Read the model definition and answer for the solid it produces. Units are mm, in the model's axes. Face numbers are marked on the shaded views. A direction names the side the tool comes from. Coordinates: 2 decimals unless noted, no trailing zeros. Order: outer loops, then holes, each group sorted by start corner. A loop starts at its lowest first (then second) coordinate and runs counter-clockwise, first axis right, second up. Notation, with made-up numbers: M 14,-35.5 L 73,-35.5 A10 ccw 73,-26.5 Z; hole C -31,37.25 d4. An arc over 180 degrees is marked long. Write each question's results on one line, items separated by ' | '.
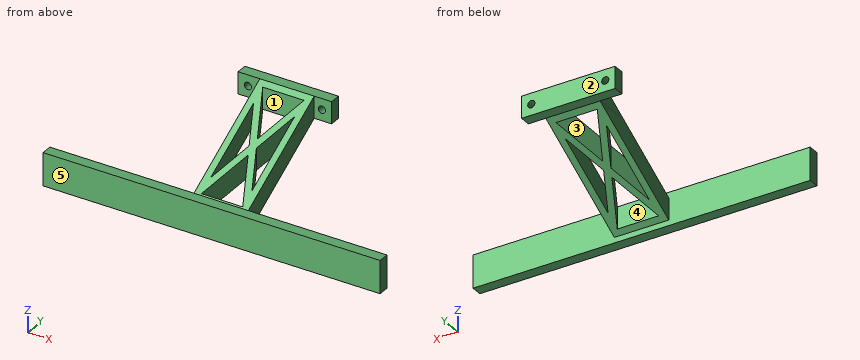
Autodesk Inventor part; units mm, degrees
ref_plane "YZ Plane" through (0, 0, 0) normal (1, 0, 0) x (0, 1, 0)
ref_plane "XZ Plane" through (0, 0, 0) normal (0, 1, 0) x (-1, 0, 0)
ref_plane "XY Plane" through (0, 0, 0) normal (0, 0, 1) x (1, 0, 0)
ref_plane "工作平面2" through (-119.683, -39.1814, 539.2089) normal (0, -1, 0) x (-0.0000021, 0, 1)
sketch "草图2" plane through (-119.683, -39.1814, 539.2089) normal (0, -1, 0) x (-0.0000021, 0, 1)
  line L0 (-31, -79.3909) -> (-41, -79.3909)
  line L1 (-41, -79.3909) -> (-41, -36.3909)
  line L2 (-41, -36.3909) -> (-31, -36.3909)
  line L3 (-31, -36.3909) -> (-31, -79.3909)
  circle A0 centre (-36, -74.8909) radius 1.65
  circle A1 centre (-36, -40.8909) radius 1.65
  point P0 (-539.2092, -119.6818)
  point P1 (0, 0)
  dimension "d0" = 10
  dimension "d1" = 43
  dimension "d2" = 5
  dimension "d3" = 4.5
extrude "拉伸1" add sketch "草图2" along normal blind 5
ref_plane "工作平面3" through (-119.683, -44.1814, 539.2089) normal (0, -1, 0) x (1, 0, 0.0000021)
sketch "草图4" plane through (-119.683, -44.1814, 539.2089) normal (0, -1, 0) x (1, 0, 0.0000021)
  line L0 (36.3909, -41) -> (79.3909, -41)
  line L1 (79.3909, -31) -> (36.3909, -31)
  line L2 (71.3909, -41) -> (46.3909, -41)
  line L3 (46.3909, -41) -> (46.3909, -31)
  line L4 (46.3909, -31) -> (71.3909, -31)
  line L5 (71.3909, -31) -> (71.3909, -41)
  line L6 (36.3909, -31) -> (36.3909, -41)
  point P0 (119.6818, -539.2092)
  point P1 (71.3909, -31)
  point P2 (46.3909, -41)
  dimension "d10" = 25
  dimension "d11" = 10
extrude "拉伸4" add sketch "草图4" along normal blind 50 contours L3 L1 L5 L0
sketch "草图5" plane through (-48.292, -94.1814, 508.2091) normal (1, 0, 0.0000021) x (0.0000021, 0, -1)
  line L0 (0, 50) -> (10, 50)
  line L1 (0, 50) -> (0, 0)
  line L2 (10, 0) -> (0, 0)
  line L3 (10, 50) -> (10, 0)
  line L4 (0, 50) -> (28.8675, 0)
  line L5 (28.8675, 0) -> (38.8675, 0)
  line L6 (38.8675, 0) -> (10, 50)
  point P0 (508.2092, 94.1814)
  point P1 (10, 32.6795)
  dimension "d29" = 30
extrude "拉伸5" add sketch "草图5" against normal blind 25 contours L6 L5 L4 L3
extrude "拉伸6" cut sketch "草图5" against normal blind 25 contours L4 L3 L2 L1
ref_plane "工作平面4" through (-40.292, -44.1814, 508.2091) normal (-0.0000021, 0, 1) x (1, 0, 0.0000021)
sketch "草图7" plane through (-40.292, -44.1814, 508.2091) normal (-0.0000021, 0, 1) x (1, 0, 0.0000021)
  line L0 (-8, 0) -> (-8, -50)
  line L1 (-33, 0) -> (-8, 0)
  line L2 (-33, -50) -> (-33, 0)
  line L3 (-8, -50) -> (-33, -50)
  line L4 (-40.6091, 5) -> (-2.3909, 5)
  line L5 (-33, 0) -> (-8, 0)
  line L6 (0, 0) -> (-8, 0)
  line L7 (0, 5) -> (0, 0)
  line L8 (0, 5) -> (-43, 5)
  line L9 (-43, 5) -> (-43, 0)
  line L10 (-33, 0) -> (-43, 0)
  line L11 (-8, 0) -> (-33, 0)
  line L12 (-33, 0) -> (-8, -50)
  line L13 (-33, -50) -> (-8, 0)
  line L14 (-31.3229, 0) -> (-8, -46.6459)
  line L15 (-33, -3.3541) -> (-9.6771, -50)
  line L16 (-33, -50) -> (-33, 0)
  line L17 (-33, -46.6459) -> (-9.6771, 0)
  line L18 (-8, -50) -> (-8, 0)
  line L19 (-8, -3.3541) -> (-31.3229, -50)
  line L20 (-30, 0) -> (-30, -50)
  line L21 (-11, -50) -> (-11, 0)
  line L22 (-30, -47.3541) -> (-11, -47.3541)
  line L23 (-30, -2.6459) -> (-11, -2.6459)
  point P0 (40.291, 44.1814)
  point P1 (-33, -46.6459)
  point P2 (-22.1771, -25)
  point P3 (-20.5, -28.3541)
  point P4 (-8, -3.3541)
  point P5 (-18.8229, -25)
  point P6 (-20.5, -21.6459)
  point P7 (-9.6771, 0)
  point P8 (-31.3229, 0)
  point P9 (-11, -40.6459)
  point P10 (-11, -9.3541)
  point P11 (-30, -9.3541)
  point P12 (-30, -40.6459)
  point P13 (-11, -2.6459)
  point P14 (-11, 0)
  point P15 (-30, 0)
  point P16 (-30, -2.6459)
  point P17 (-11, -47.3541)
  point P18 (-30, -47.3541)
  dimension "d44" = 1.5
  dimension "d45" = 1.5
  dimension "d47" = 3
  dimension "d48" = 3
extrude "拉伸8" cut sketch "草图7" against normal blind 50 contours L21 L14 L19 | L17 L14 L23 | L22 L19 L15 | L17 L20 L15
ref_plane "工作平面5" through (-48.2919, -94.1814, 469.3416) normal (0, -1, 0) x (1, 0, 0.0000021)
sketch "草图8" plane through (-48.2919, -94.1814, 469.3416) normal (0, -1, 0) x (1, 0, 0.0000021)
  line L0 (0, 10) -> (0, 0) construction
  line L1 (-25, 0) -> (-25, 10) construction
  line L2 (-90, -2.5) -> (65, -2.5)
  line L3 (65, -2.5) -> (65, 12.5)
  line L4 (65, 12.5) -> (-90, 12.5)
  line L5 (-90, 12.5) -> (-90, -2.5)
  line L6 (0, 10) -> (-25, 10)
  line L7 (0, 0) -> (-25, 0)
  line L8 (0, 10) -> (-25, 10)
  line L9 (0, 0) -> (-25, 0)
  point P0 (48.291, -469.3417)
  dimension "d40" = 155
  dimension "d41" = 65
  dimension "d49" = 15
  dimension "d50" = 2.5
extrude "拉伸9" add sketch "草图8" along normal blind 5
properties part number "起落架 新"
(1) The part is cut by section A-A, the plane x = -65. Write down the section's boundary in (y, z), then the cut area to 3 significant figures.
Conclusion:
outline: M -99.18,466.84 L -94.18,466.84 L -94.18,469.34 L -91.54,470.87 L -91.54,480.87 L -94.18,479.34 L -94.18,481.84 L -99.18,481.84 Z; M -80.95,476.98 L -74.24,480.85 L -74.24,490.85 L -80.95,486.98 Z; M -64.12,486.7 L -57.41,490.57 L -57.41,500.57 L -64.12,496.7 Z; M -46.83,496.68 L -44.18,498.21 L -39.18,498.21 L -39.18,508.21 L -44.18,508.21 L -46.83,506.68 Z | area: 312 mm²
(2) The part is cut by section B-B, the plane y = -82. Write down the section's boundary in (x, z).
Conclusion:
outline: M -73.29,476.37 L -70.29,476.37 L -70.29,486.37 L -73.29,486.37 Z; M -68.88,476.37 L -65.52,476.37 L -65.52,486.37 L -68.88,486.37 Z; M -56.06,476.37 L -52.71,476.37 L -52.71,486.37 L -56.06,486.37 Z; M -51.29,476.37 L -48.29,476.37 L -48.29,486.37 L -51.29,486.37 Z
(3) Given pin 1 (6 mm diameter, centred on x = -70.5, z = 479.5, fed in from +Y); pin 2 (1.5 mm diameter, centred on y = -41, z = 504, fed in from +X); pin 3 (14.5 mm diameter, centred on y = -76.5, z = 481, fed in from -X); pin 4 (4 mm diameter, centred on x = -78.79, z = 503.21, fed in from +Y), each flat-ended and moving along its own axis, determine where each tip first touches the part or whether it passes through.
Conclusion:
pin 1: y = -71.39 | pin 2: x = -40.29 | pin 3: x = -73.29 | pin 4: y = -39.18
(4) For the marked faces 4 and 5, determine the directions among +Z, -Z, +X, -X, +Y, -Y from which every point of the face is accessible in a straight line to the end or side of a thin tool.
Conclusion:
face 4: +Z, -Z | face 5: +Z, -Z, +X, -X, -Y
(5) The part is cut by section D-D, the plane y = -71. Write down the section's boundary in (x, z).
Conclusion:
outline: M -73.29,482.73 L -70.29,482.73 L -70.29,492.73 L -73.29,492.73 Z; M -63.38,482.73 L -58.21,482.73 L -58.21,492.73 L -63.38,492.73 Z; M -51.29,482.73 L -48.29,482.73 L -48.29,492.73 L -51.29,492.73 Z
(6) The part is cut by section C-C, the plane y = -88. Write down the section's boundary in (x, z).
Conclusion:
outline: M -73.29,472.91 L -68.52,472.91 L -68.52,482.91 L -73.29,482.91 Z; M -53.06,472.91 L -48.29,472.91 L -48.29,482.91 L -53.06,482.91 Z
(7) The mould has two halves that part along X. Classify the marked faces 1, 2 and 3: pulls with the +X half, pulls with the -X half, needs draft (parallel to the pull), parting line crosses it, or undercut.
Conclusion:
face 1: undercut | face 2: needs draft | face 3: undercut
(8) Straight lines are drawn through the part: line 1 (X direction, y = -71.5, z = 488.5); line 2 (X direction, y = -84, z = 482.5); line 3 (X direction, y = -60, z = 494). For each, find the intervals that lie inside material, in ascending order.
Conclusion:
line 1: -73.29 to -70.29, -63.63 to -57.96, -51.29 to -48.29 | line 2: -73.29 to -70.29, -69.88 to -66.52, -55.06 to -51.71, -51.29 to -48.29 | line 3: -73.29 to -70.29, -67.06 to -63.71, -57.88 to -54.52, -51.29 to -48.29
